Verification items for this drawing (mm, ordinates from the low corner). Coordinates: 2 decimals unless noted, no trailing zeros. Order: outer loops, then holes, each group sorted by start corner. A loop starts at its lowest first (then second) coordinate and runs counter-clockwise, first axis right, second up.
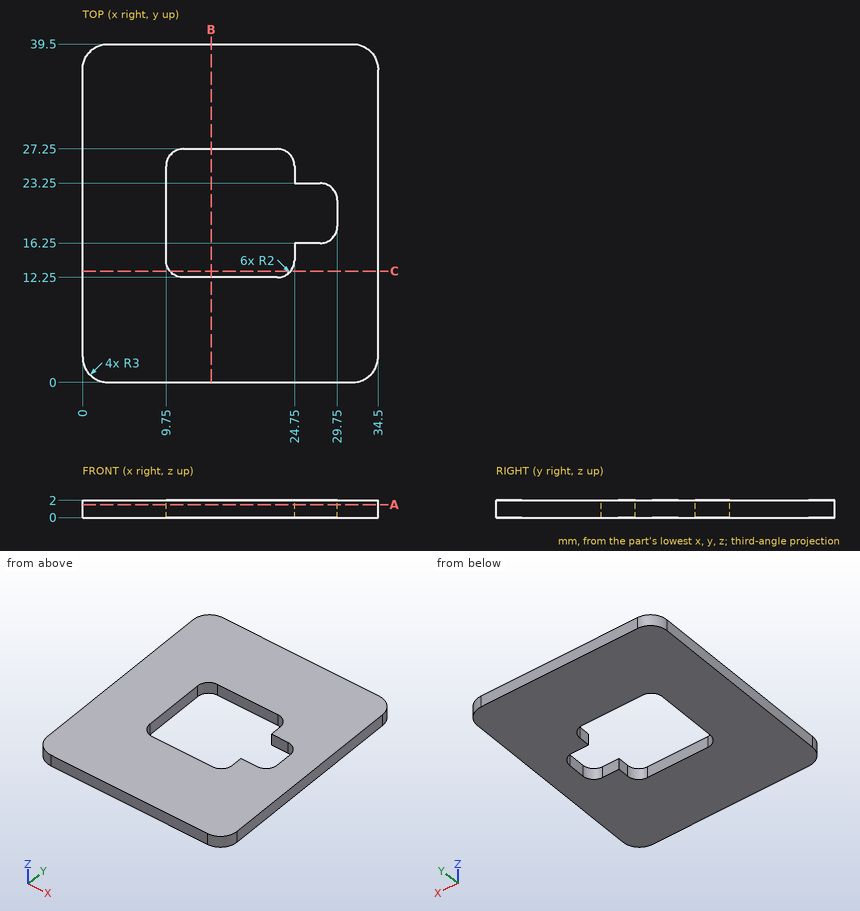
Item 1: Sectioned sample at B-B (x = 15). Record the cut outline in (y, z).
Item 2: Thickness scan on line 1 along Y through (x, z) = (25, 0.9); line 2 along Y through (x, z) = (16, 1.7); line 3 along X through (y, z) = (14.5, 0.7). Record the ranges inside material, lowest first.
Item 3: Sectioned sample at C-C (y = 13). Record the cut outline in (x, z), and give its area (3 significant figures).
Item 4: Sectioned sample at A-A (z = 1.5). Record the cut outline in (x, y), and give its area (3 significant figures).
Geometry check:
1. outline: (0, 0) - (12.25, 0) - (12.25, 2) - (0, 2) - close; (27.25, 0) - (39.5, 0) - (39.5, 2) - (27.25, 2) - close
2. line 1: y = 0 to 16.25, 23.25 to 39.5
2. line 2: y = 0 to 12.25, 27.25 to 39.5
2. line 3: x = 0 to 9.75, 24.75 to 34.5
3. outline: (0, 0) - (10.19, 0) - (10.19, 2) - (0, 2) - close; (24.31, 0) - (34.5, 0) - (34.5, 2) - (24.31, 2) - close
3. area: 40.8 mm2
4. outline: (0, 3) arc R3 ccw to (3, 0) - (31.5, 0) arc R3 ccw to (34.5, 3) - (34.5, 36.5) arc R3 ccw to (31.5, 39.5) - (3, 39.5) arc R3 ccw to (0, 36.5) - close; hole (9.75, 14.25) arc R2 ccw to (11.75, 12.25) - (22.75, 12.25) arc R2 ccw to (24.75, 14.25) - (24.75, 16.25) - (27.75, 16.25) arc R2 ccw to (29.75, 18.25) - (29.75, 21.25) arc R2 ccw to (27.75, 23.25) - (24.75, 23.25) - (24.75, 25.25) arc R2 ccw to (22.75, 27.25) - (11.75, 27.25) arc R2 ccw to (9.75, 25.25) - close
4. area: 1,100 mm2
